Answer from the drawing. Dimensions are ordinates in mm from the lowest x, y and z of the part. A direction names the side the tool comes from. Give positions to 0.01 mm unless a question says otherwise; leave off trailing zeros. Order: outer loops, then holes, each group sorted by start corner. A loop starts at its lowest first (then second) coordinate and runs counter-clockwise, first axis right, second up. Notation, with made-up numbers: (89, -24.75) - (131, -24.75) arc R13 cw to (131, -17.75) - close; hole circle Ø7 at (-6.75, 50). An arc over 180 degrees is marked (long way). Use a Markdown table: item, result. Add a question column.
1) Find section D-D, the plane y = 10. Determine the outline of the cut face in (x, z).
2) Straight lines are drawn through the part: line 1 (X direction, y = 2.5, z = 11); line 2 (Z direction, x = 10, y = 14.75). For each, find the intervals that lie inside material, in ascending order.
3) Find section B-B, the plane z = 11.5. Determine the outline of the cut face in (x, y).
4) The mould has two halves that part along Y. Classify the marked faces 1, 2 and 3: released by +Y, released by -Y, zero draft, split by the parting line, or undercut.
5) Find section A-A, the plane x = 10. Determine the outline of the cut face in (y, z), plus the area to 3 significant figures.
6) For the marked faces 4 and 5, determine the directions among +Z, -Z, +X, -X, +Y, -Y from which every point of the face is accessible in a straight line to the end or side of a thin tool.
7) Find section C-C, the plane z = 3.25. Determine the outline of the cut face in (x, y), plus the area to 3 significant figures.
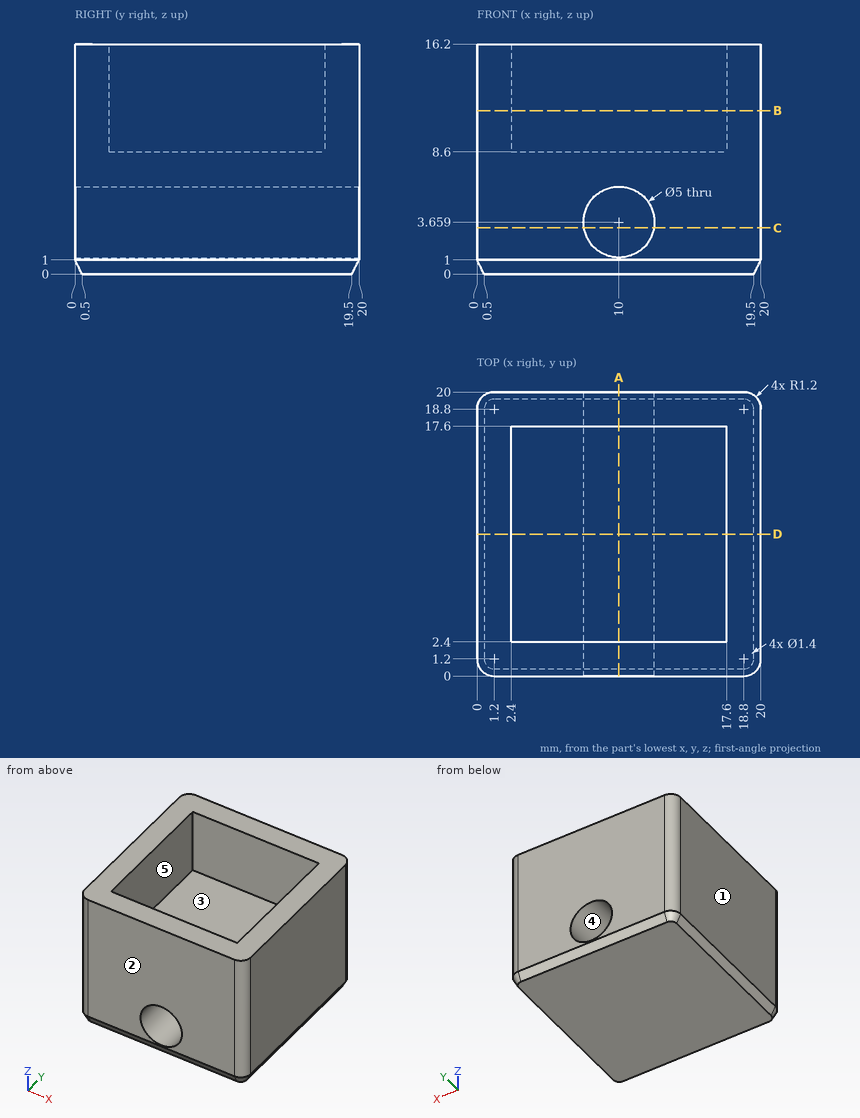
The answers:
| question | item | result |
|---|---|---|
| 1 | outline | (0, 1) - (0.5, 0) - (19.5, 0) - (20, 1) - (20, 16.2) - (17.6, 16.2) - (17.6, 8.6) - (2.4, 8.6) - (2.4, 16.2) - (0, 16.2) - close; hole circle Ø5 at (10, 3.66) |
| 2 | line 1 | 0 to 2.4, 17.6 to 20 |
| 2 | line 2 | 0 to 1.16, 6.16 to 8.6 |
| 3 | outline | (0, 1.2) arc R1.2 ccw to (1.2, 0) - (18.8, 0) arc R1.2 ccw to (20, 1.2) - (20, 18.8) arc R1.2 ccw to (18.8, 20) - (1.2, 20) arc R1.2 ccw to (0, 18.8) - close; hole (2.4, 2.4) - (17.6, 2.4) - (17.6, 17.6) - (2.4, 17.6) - close |
| 4 | face 1 | zero draft |
| 4 | face 2 | released by -Y |
| 4 | face 3 | undercut |
| 5 | outline | (0, 1) - (0.5, 0) - (19.5, 0) - (20, 1) - (20, 1.16) - (0, 1.16) - close; (0, 6.16) - (20, 6.16) - (20, 16.2) - (17.6, 16.2) - (17.6, 8.6) - (2.4, 8.6) - (2.4, 16.2) - (0, 16.2) - close |
| 5 | area | 108 mm2 |
| 6 | face 4 | +Y, -Y |
| 6 | face 5 | +Z |
| 7 | outline | (0, 1.2) arc R1.2 ccw to (1.2, 0) - (7.53, 0) - (7.53, 20) - (1.2, 20) arc R1.2 ccw to (0, 18.8) - close; (12.47, 0) - (18.8, 0) arc R1.2 ccw to (20, 1.2) - (20, 18.8) arc R1.2 ccw to (18.8, 20) - (12.47, 20) - close |
| 7 | area | 300 mm2 |
